```python
from build123d import *

# Parameters (mm, degrees)
SKETCH_1_W                  = 40
SKETCH_1_H                  = 47.1
EXTRUDE_1_DEPTH             = 5
HOLE_WIZARD_M4_1_AT_2_COUNT = 2
HOLE_WIZARD_M4_1_AT_2_PITCH = 32
SKETCH_5_R                  = 2.1
CUT_EXTRUDE_M5_DEPTH        = 25
SKETCH_6_R                  = 6
EXTRUDE_1739_DEPTH          = 10
FILLET_1_R                  = 5
SKETCH_7_W                  = 24
SKETCH_7_H                  = 27.1
CUT_EXTRUDE_1_DEPTH         = 10
FILLET_2_R                  = 3
F_4_0MM_1_AT_2_COUNT        = 2
F_4_0MM_1_AT_2_PITCH        = 15
CUT_EXTRUDE_3_DEPTH         = 10
FILLET_3_R                  = 2


with BuildPart() as part:
    # 草图1 → 凸台-拉伸1 (new, symmetric)
    with BuildSketch(Plane.XY):
        Rectangle(SKETCH_1_W, SKETCH_1_H)
    extrude(amount=EXTRUDE_1_DEPTH, both=True)

    # 草图4 → M4 螺纹孔1 (revolve, cut)
    with BuildSketch(Plane(origin=(-16, 23.55, 0), x_dir=(0, 0, 1), z_dir=(1, 0, 0))):
        Polygon((0, 0), (0, 11.091420021), (1.65, 10.1), (1.65, 0), align=None)
    hole_wizard_m4_1 = revolve(axis=Axis((-16, 29.9, 0), (0, -1, 0)), mode=Mode.SUBTRACT)

    # M4 螺纹孔1 at 2: M4 螺纹孔1 ×2
    with Locations(*[(i * HOLE_WIZARD_M4_1_AT_2_PITCH, 0, 0) for i in range(1, HOLE_WIZARD_M4_1_AT_2_COUNT)]):
        add(hole_wizard_m4_1, mode=Mode.SUBTRACT)

    # 镜向1: M4 螺纹孔1 across plane
    add(hole_wizard_m4_1.mirror(Plane.ZX), mode=Mode.SUBTRACT)

    # 镜向1 copy 1 sketch → 镜向1 copy 1 (revolve, cut)
    with BuildSketch(Plane(origin=(16, -23.55, 0), x_dir=(0, 0, 1), z_dir=(1, 0, 0))):
        Polygon((0, 0), (0, -11.091420021), (1.65, -10.1), (1.65, 0), align=None)
    revolve(axis=Axis((16, -29.9, 0), (0, -1, 0)), mode=Mode.SUBTRACT)

    # 草图5 → M5螺纹孔 (cut, symmetric)
    with BuildSketch(Plane.XY.offset(5)):
        with Locations(Location((0, 0, 0), (0, 0, 180))):
            Circle(SKETCH_5_R)
    extrude(amount=CUT_EXTRUDE_M5_DEPTH, both=True, mode=Mode.SUBTRACT)

    # 草图6 → Extrude 1739 (add)
    with BuildSketch(Plane.XY.offset(5)):
        with BuildLine():
            Line((42.499604204, 7.599472273), (20, 15))
            Line((20, 15), (20, -15))
            Line((20, -15), (42.499604204, -7.599472273))
            ThreePointArc((42.499604204, -7.599472273), (48, 0), (42.499604204, 7.599472273))
        make_face()
        with Locations((40, 0)):
            Circle(SKETCH_6_R, mode=Mode.SUBTRACT)
    extrude(amount=-EXTRUDE_1739_DEPTH)

    # 圆角1
    fillet_1_edges = [part.edges().sort_by_distance(p)[0] for p in [
        (20, -15, 0),
        (20, 15, 0),
    ]]
    fillet(fillet_1_edges, radius=FILLET_1_R)

    # 草图7 → 切除-拉伸1 (cut)
    with BuildSketch(Plane.XY.offset(5)):
        with Locations((-20, 0)):
            Rectangle(SKETCH_7_W, SKETCH_7_H)
    extrude(amount=-CUT_EXTRUDE_1_DEPTH, mode=Mode.SUBTRACT)

    # 圆角2
    fillet_2_edges = [part.edges().sort_by_distance(p)[0] for p in [
        (-8, -13.55, 0),
        (-8, 13.55, 0),
    ]]
    fillet(fillet_2_edges, radius=FILLET_2_R)

    # 草图11 → Ø4.0mm 暗销孔1 (revolve, cut)
    with BuildSketch(Plane(origin=(-7.5, 23.55, 0), x_dir=(0, 0, 1), z_dir=(1, 0, 0))):
        Polygon((0, 0), (0, 6.201721238), (2, 5), (2, 0), align=None)
    f_4_0mm_1 = revolve(axis=Axis((-7.5, 29.9, 0), (0, -1, 0)), mode=Mode.SUBTRACT)

    # Ø4.0mm 暗销孔1 at 2: Ø4.0mm 暗销孔1 ×2
    with Locations(*[(i * F_4_0MM_1_AT_2_PITCH, 0, 0) for i in range(1, F_4_0MM_1_AT_2_COUNT)]):
        add(f_4_0mm_1, mode=Mode.SUBTRACT)

    # 镜向3: Ø4.0mm 暗销孔1 across plane
    add(f_4_0mm_1.mirror(Plane.ZX), mode=Mode.SUBTRACT)

    # 镜向3 copy 1 sketch → 镜向3 copy 1 (revolve, cut)
    with BuildSketch(Plane(origin=(7.5, -23.55, 0), x_dir=(0, 0, 1), z_dir=(1, 0, 0))):
        Polygon((0, 0), (0, -6.201721238), (2, -5), (2, 0), align=None)
    revolve(axis=Axis((7.5, -29.9, 0), (0, -1, 0)), mode=Mode.SUBTRACT)

    # 草图12 → 切除-拉伸3 (cut)
    with BuildSketch(Plane.XY.offset(5)):
        with BuildLine():
            Line((8, 13.683494171), (8, -13.683494171))
            Line((8, -13.683494171), (32.876894011, -5.501032727))
            ThreePointArc((32.876894011, -5.501032727), (31, 0), (32.876894011, 5.501032727))
            Line((32.876894011, 5.501032727), (8, 13.683494171))
        make_face()
    extrude(amount=-CUT_EXTRUDE_3_DEPTH, mode=Mode.SUBTRACT)

    # 圆角3
    fillet_3_edges = [part.edges().sort_by_distance(p)[0] for p in [
        (8, 13.683494171, 0),
        (32.876894011, 5.501032727, 0),
        (32.876894011, -5.501032727, 0),
        (8, -13.683494171, 0),
    ]]
    fillet(fillet_3_edges, radius=FILLET_3_R)


solid = part.part
```
Work out the finished part from the listing and answer in its coordinate system (mm). A direction names the side the tool comes from. Round coordinates to 2 decimals unless told otherwise and drop trailing zeros. Write each loop counter-clockwise with the first axis right and the second up, starting at its lowest first coordinate (ties: lowest second). Pieces come first, ordered by that corner, then holes. Notation, with made-up numbers: (51.5, 26.25) -> (71.5, 26.25) arc R16 ccw to (71.5, 52.25) -> close; hole circle Ø9 at (-25.75, 59.25). An arc over 180 degrees is marked (long way). Write each question's results on one line, items separated by ' | '.
Q1. Flat-ended cylindrical pins translate along their axes: P1, Ø1.5, axis at y = 4, z = 1.5, coming from the +X side; P2, Ø4, axis at y = 20.5, z = -1, coming from the +X side; P3, Ø2.5, axis at x = 7.5, z = 0, coming from the +Y side; P4, Ø3.5, axis at x = 0, y = 0, coming from the -Z side. Find the tip coordinate at first contact, or state that the pin passes through.
Data:
P1: x = 47.31 | P2: x = 20 | P3: y = 18.1 | P4: through
Q2. Section A-A, the plane y = 0 is taken. Write down the section's boundary in (x, z), then the cut area to 3 significant figures.
Data:
outline: (-8, -5) -> (-2.1, -5) -> (-2.1, 5) -> (-8, 5) -> close; (2.1, -5) -> (8, -5) -> (8, 5) -> (2.1, 5) -> close; (31, -5) -> (34, -5) -> (34, 5) -> (31, 5) -> close; (46, -5) -> (48, -5) -> (48, 5) -> (46, 5) -> close | area: 168 mm^2
Q3. Section D-D, the plane x = 41 is taken. Write down the section's boundary in (y, z), then the cut area to 3 significant figures.
Data:
outline: (-8.09, -5) -> (-5.92, -5) -> (-5.92, 5) -> (-8.09, 5) -> close; (5.92, -5) -> (8.09, -5) -> (8.09, 5) -> (5.92, 5) -> close | area: 43.5 mm^2
Q4. Determine the mould class of faces 4 (the conical face through (-7.19, 17.56, 0.16)), 5 (the flat face through (32.835, -10.778, 0.07)), 6 (the flat face through (6, 0, -5)) for opening direction Z: released by +Z, released by -Z, zero draft, split by the parting line, or undercut.
Data:
face 4: undercut | face 5: zero draft | face 6: released by -Z
Q5. Straight lines are drawn through the part: line 1 along X through (y, z) = (-22, 0); line 2 along X through (y, z) = (17, -0.25); line 3 along X through (y, z) = (18, 0.25). For each, find the intervals that lie inside material, in ascending order. Write a range as [from, to].
Data:
line 1: [-20, -17.65], [-14.35, -9.5], [-5.5, 5.5], [9.5, 14.35], [17.65, 20] | line 2: [-20, -17.63], [-14.37, 14.37], [17.63, 20.27] | line 3: [-20, -17.63], [-14.37, -8.56], [-6.44, 6.44], [8.56, 14.37], [17.63, 20.04]
Q6. Section B-B, the plane x = -16 is taken. Write down the section's boundary in (y, z).
Data:
outline: (-23.55, -5) -> (-13.55, -5) -> (-13.55, -1.65) -> (-23.55, -1.65) -> close; (-23.55, 1.65) -> (-13.55, 1.65) -> (-13.55, 5) -> (-23.55, 5) -> close; (13.55, -5) -> (23.55, -5) -> (23.55, -1.65) -> (13.55, -1.65) -> close; (13.55, 1.65) -> (23.55, 1.65) -> (23.55, 5) -> (13.55, 5) -> close
Q7. Section C-C, the plane z = -3 is taken. Write down the section's boundary in (x, y).
Data:
outline: (-20, -23.55) -> (20, -23.55) -> (20, -18.62) arc R5 cw to (23.44, -13.87) -> (42.5, -7.6) arc R8 ccw to (42.5, 7.6) -> (23.44, 13.87) arc R5 cw to (20, 18.62) -> (20, 23.55) -> (-20, 23.55) -> (-20, 13.55) -> (-11, 13.55) arc R3 cw to (-8, 10.55) -> (-8, -10.55) arc R3 cw to (-11, -13.55) -> (-20, -13.55) -> close; hole circle Ø4.2 at (0, 0); hole (8, -10.92) arc R2 ccw to (10.62, -12.82) -> (30.53, -6.27) arc R2 ccw to (31.74, -3.58) arc R9 cw to (31.74, 3.58) arc R2 ccw to (30.53, 6.27) -> (10.62, 12.82) arc R2 ccw to (8, 10.92) -> close; hole circle Ø12 at (40, 0)
Q8. Which of the six approach directions +Z, -Z, +X, -X, +Y, -Y give full straight-line access (tool end or side, diameter ignored) to faces 1 (the cylindrical face through (31.721, -5.213, -0.07)), 2 (the cylindrical face through (-9.483, -21.085, -0.26)), 3 (the flat face through (20, 21, 0))?
Data:
face 1: +Z, -Z | face 2: -Y | face 3: +Z, -Z, +X, +Y
